Answer from the drawing. Dimensions are ordinates in mm from the lowest x, y and z of the part. A direction names the side the tool comes from. Coordinates: 2 decimals unless noted, no trailing zeros. Write each loop counter-clockwise with the first axis right and the second up, starting at its lowest first coordinate (ties: lowest second). Pieces come first, ordered by that corner, then holes. Notation, with made-up numbers: (20, 77.5) - (36, 77.5) arc R31 ccw to (36, 110.5) - close; hole circle Ø4 at (75, -21.75). An arc over 180 degrees is marked (long way). Use a Markdown table: item, result.
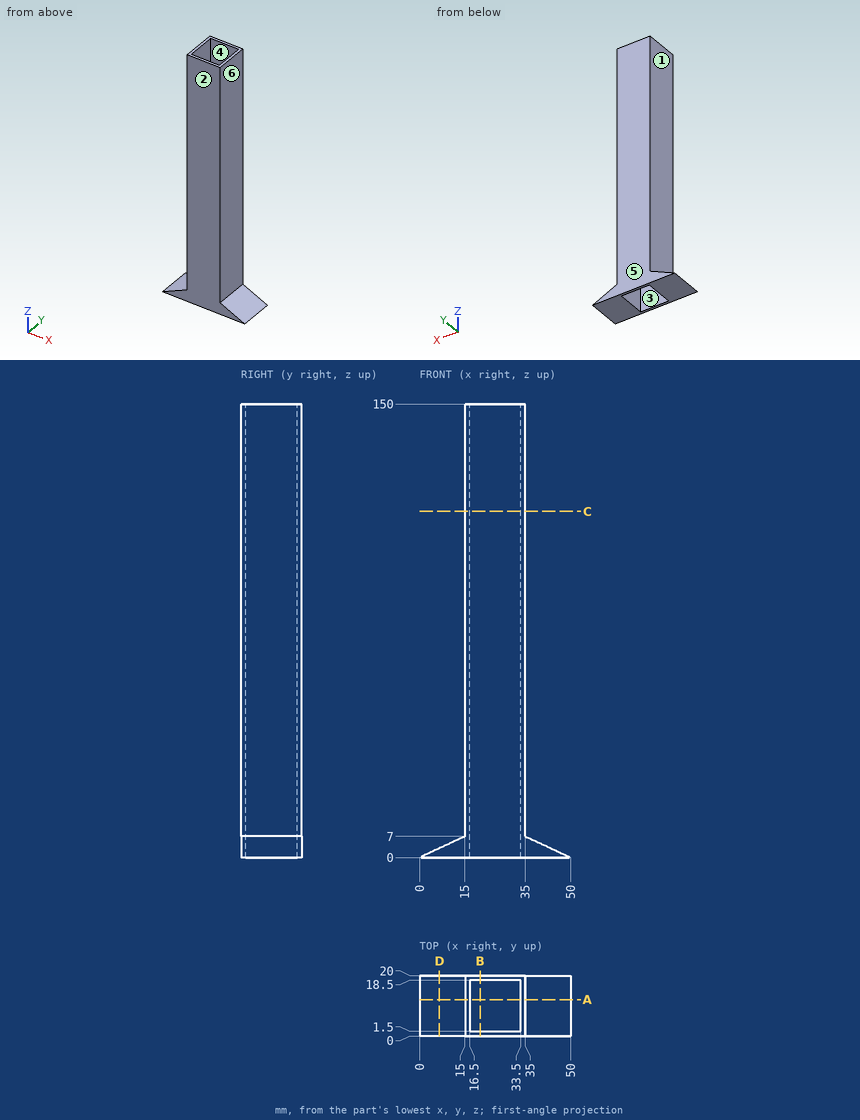
(1) Straight lines are drawn through the part: L1, parallel to Y at x = 27, z = 20; L2, parallel to X at y = 5.5, z = 11.5; L3, parallel to X at y = 1, z = 46. For each, find the intervals that lie inside material, in ascending order.
Report:
| item | result |
|---|---|
| L1 | y = 0 to 1.5, 18.5 to 20 |
| L2 | x = 15 to 16.5, 33.5 to 35 |
| L3 | x = 15 to 35 |
(2) A cutting plane is placed at D-D, the plane x = 6.5. Write down the section's boundary in (y, z), and give its area (3 significant figures).
Report:
| item | result |
|---|---|
| outline | (0, 0) - (20, 0) - (20, 3.03) - (0, 3.03) - close |
| area | 60.7 mm² |
(3) A cutting plane is placed at B-B, the plane x = 20. Write down the section's boundary in (y, z).
Report:
| item | result |
|---|---|
| outline | (0, 0) - (1.5, 0) - (1.5, 150) - (0, 150) - close; (18.5, 0) - (20, 0) - (20, 150) - (18.5, 150) - close |
(4) For the marked faces 1, 2 and 3, determine the directions among +Z, -Z, +X, -X, +Y, -Y from which every point of the face is accessible in a straight line to the end or side of a thin tool.
Report:
| item | result |
|---|---|
| face 1 | +Z, -X, +Y, -Y |
| face 2 | +Z, -Z, +X, -X, -Y |
| face 3 | +Z, -Z |
(5) Each of these flat-tipped pins is pushed along its axis until it touches: P1, Ø4, axis at x = 24.5, y = 15.5, coming from the +Z side; P2, Ø1, axis at y = 15, z = 78, coming from the -X side. Where does it stop, or does it pass through?
Report:
| item | result |
|---|---|
| P1 | passes through |
| P2 | stops at x = 15 |
(6) A cutting plane is placed at C-C, the plane z = 114.5. Write down the section's boundary in (x, y), and give its area (3 significant figures).
Report:
| item | result |
|---|---|
| outline | (15, 0) - (35, 0) - (35, 20) - (15, 20) - close; hole (16.5, 1.5) - (33.5, 1.5) - (33.5, 18.5) - (16.5, 18.5) - close |
| area | 111 mm² |
(7) The mould has two halves that part along Y. Classify the marked faces 4, 5 and 6: pulls with the +Y half, pulls with the -Y half, needs draft (parallel to the pull), parting line crosses it, or undercut.
Report:
| item | result |
|---|---|
| face 4 | undercut |
| face 5 | pulls with the +Y half |
| face 6 | needs draft |
(8) A cutting plane is placed at A-A, the plane y = 12. Write down the section's boundary in (x, z), and give its area (3 significant figures).
Report:
| item | result |
|---|---|
| outline | (0, 0) - (16.5, 0) - (16.5, 150) - (15, 150) - (15, 7) - close; (33.5, 0) - (50, 0) - (35, 7) - (35, 150) - (33.5, 150) - close |
| area | 555 mm² |
